Verification items for this drawing (mm, ordinates from the low corner). A direction names the side the tool comes from. Coordinates: 2 decimals unless noted, no trailing zeros. Order: outer loops, then holes, each group sorted by start corner. A loop starts at its lowest first (then second) coordinate and runs counter-clockwise, first axis right, second up. Notation, with made-up numbers: M -32,89.25 L -18,89.25 A16 cw -18,109.25 Z; hole C -25.5,20 d1. An arc over 180 degrees is marked long. Write item = value, one per line.
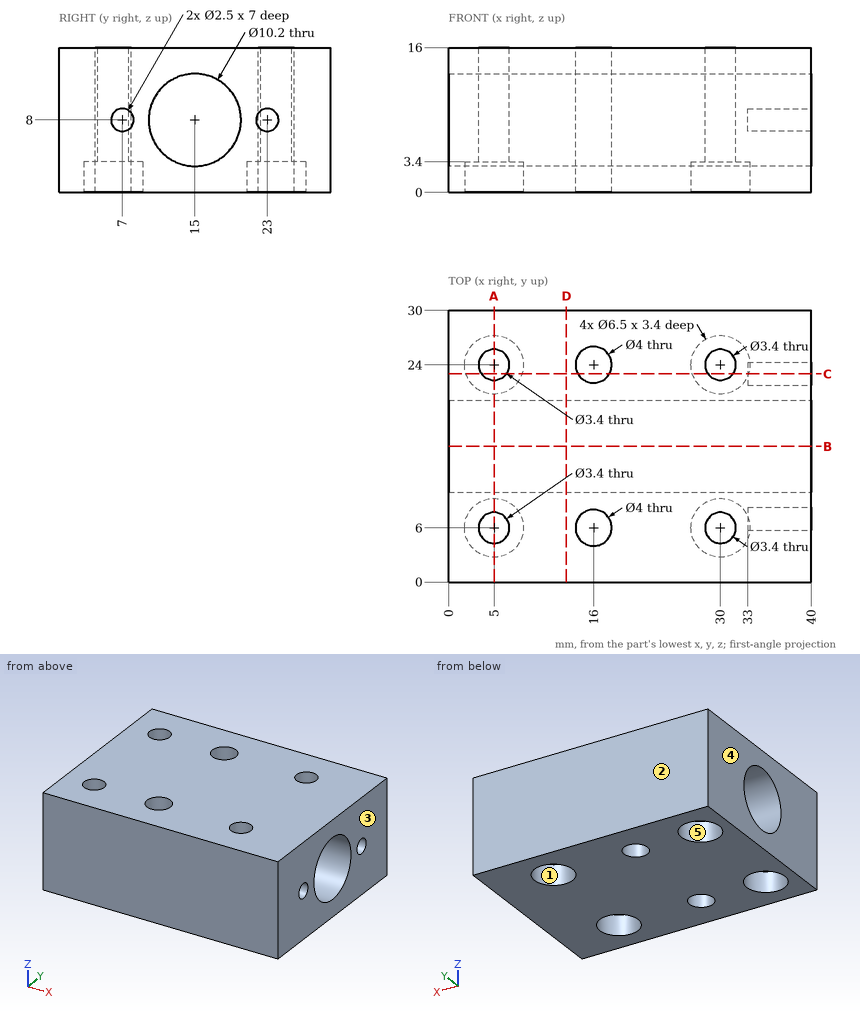
Item 1: Sectioned sample at B-B, the plane y = 15. Enter the section's corners in (x, z).
Report:
outline = M 0,0 L 40,0 L 40,2.9 L 0,2.9 Z; M 0,13.1 L 40,13.1 L 40,16 L 0,16 Z
Item 2: Tool access check on the marked faces 4 and 5. Record the directions out of +Z, -Z, +X, -X, +Y, -Y that give a thin tool (end or side, any length) a straight path to the whole face; none if there is none.
Report:
face_4 = +Z, -Z, -X, +Y, -Y
face_5 = -Z
Item 3: Sectioned sample at A-A, the plane x = 5. Enter the section's corners in (y, z), then the cut area to 3 significant figures.
Report:
outline = M 0,0 L 2.75,0 L 2.75,3.4 L 4.3,3.4 L 4.3,16 L 0,16 Z; M 7.7,3.4 L 9.25,3.4 L 9.25,0 L 20.75,0 L 20.75,3.4 L 22.3,3.4 L 22.3,16 L 7.7,16 Z; M 25.7,3.4 L 27.25,3.4 L 27.25,0 L 30,0 L 30,16 L 25.7,16 Z; hole C 15,8 d10.2
area = 268 mm^2
Item 4: Scan lines: L1, parallel to Y at x = 5, z = 13.75; L2, parallel to Y at x = 5, z = 0.85; L3, parallel to Y at x = 38.25, z = 8. Record each from-to range of solid material in increasing order. Write a range as from..to.
Report:
L1 = 0..4.3, 7.7..22.3, 25.7..30
L2 = 0..2.75, 9.25..20.75, 27.25..30
L3 = 0..5.75, 8.25..9.9, 20.1..21.75, 24.25..30
Item 5: Gauge pin test, flat ends, axial feed: pin 1 (0.8 mm diameter, centred on y = 23, z = 8, fed in from +X); pin 2 (6 mm diameter, centred on x = 5, y = 24, fed in from -Z). Record the tip position at first contact, or that the pin passes through.
Report:
pin_1 = 33
pin_2 = 3.4
Item 6: Sectioned sample at C-C, the plane y = 23. Enter the section's corners in (x, z).
Report:
outline = M 0,0 L 1.91,0 L 1.91,3.4 L 3.63,3.4 L 3.63,16 L 0,16 Z; M 6.37,3.4 L 8.09,3.4 L 8.09,0 L 14.27,0 L 14.27,16 L 6.37,16 Z; M 17.73,0 L 26.91,0 L 26.91,3.4 L 28.63,3.4 L 28.63,16 L 17.73,16 Z; M 31.37,3.4 L 33.09,3.4 L 33.09,0 L 40,0 L 40,6.75 L 33,6.75 L 33,9.25 L 40,9.25 L 40,16 L 31.37,16 Z
Item 7: Release check for a two-part mould opening along Y. For the marked faces 1, 2 and 3 record: pulls with the +Y half, pulls with the -Y half, needs draft (parallel to the pull), parting line crosses it, or undercut.
Report:
face_1 = undercut
face_2 = pulls with the +Y half
face_3 = needs draft
Item 8: Sectioned sample at D-D, the plane x = 13. Enter the section's corners in (y, z), then the cut area to 3 significant figures.
Report:
outline = M 0,0 L 30,0 L 30,16 L 0,16 Z; hole C 15,8 d10.2
area = 398 mm^2
